```python
from build123d import *

# Parameters (mm, degrees)
SKETCH_1_W      = 20
SKETCH_1_H      = 52.5
SKETCH_1_R      = 3.1
EXTRUDE_1_DEPTH = 2
CHAMFER_1_SIZE  = 4
CHAMFER_2_SIZE  = 3


with BuildPart() as part:
    # 草图1 → 凸台-拉伸1 (new, symmetric)
    with BuildSketch(Plane.XY):
        Rectangle(SKETCH_1_W, SKETCH_1_H)
        with Locations((0, 16.25)):
            Circle(SKETCH_1_R, mode=Mode.SUBTRACT)
        with Locations((0, -3.75)):
            Circle(SKETCH_1_R, mode=Mode.SUBTRACT)
    extrude(amount=EXTRUDE_1_DEPTH, both=True)

    # 倒角1
    chamfer_1_edges = [part.edges().sort_by_distance(p)[0] for p in [
        (-10, 26.25, 0),
        (10, 26.25, 0),
        (10, -26.25, 0),
        (-10, -26.25, 0),
    ]]
    chamfer(chamfer_1_edges, length=CHAMFER_1_SIZE)

    # 倒角2
    chamfer_2_edges = [part.edges().sort_by_distance(p)[0] for p in [
        (-3.1, 16.25, 2),
        (-3.1, -3.75, 2),
    ]]
    chamfer(chamfer_2_edges, length=CHAMFER_2_SIZE)


solid = part.part
```
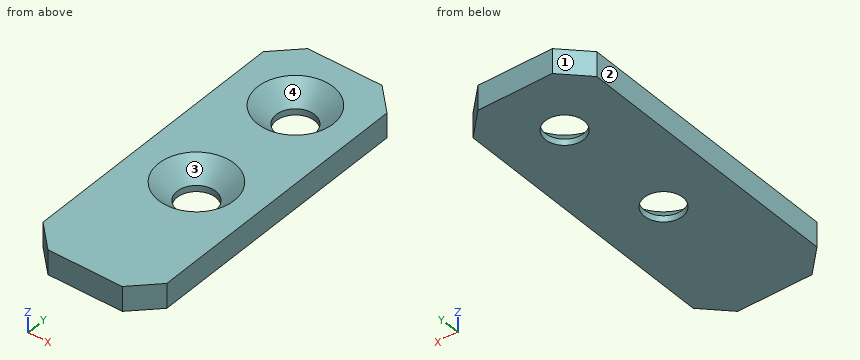
Build history of the part. All positions in model axes, mm. Face numbers are marked on the shaded views. Coordinates: 2 decimals unless noted, no trailing zeros. Order: outer loops, then holes, each group sorted by start corner. A loop starts at its lowest first (then second) coordinate and runs counter-clockwise, first axis right, second up. Notation, with made-up numbers: (57, -3.75) -> (101, -3.75) arc R5 ccw to (101, 4.25) -> close; hole circle Ø9 at (-17, -29). An arc over 180 degrees is marked (long way). Answer in a Markdown table with one row per item. Add a question column.
Q1. Band-saw the part on B-B, the plane x = 0. List the corners of the cut face in (y, z).
Q2. Wall check: line 1 along Y through (x, z) = (0, -1.8); line 2 along Y through (x, z) = (1.5, 0.85); line 3 along X through (y, z) = (17, -1.35). Give the ranges that are in metal, low to high. Write a range as [from, to].
Q3. Drop a flat-ended pin along its axis: pin 1 (2 mm diameter, centred on x = 7.5, z = 0, fed in from -Y). Give the stop position or say it passes through.
Q4. Band-saw the part on A-A, the plane y = 16.25. List the corners of the cut face in (x, z).
Q5. Band-saw the part on D-D, the plane x = -7.25. List the corners of the cut face in (y, z).
Q6. Band-saw the part on C-C, the plane z = 1. List the corners of the cut face in (x, y).
Q7. Mould opens along Y. For the marked faces 1, 2, 3 and 4 say: +Y half, -Y half, draft (parallel to the pull), parting line (faces both ways), or undercut.
Answers follow:
| question | item | result |
|---|---|---|
| 1 | outline | (-26.25, -2) -> (-6.85, -2) -> (-6.85, -1) -> (-9.85, 2) -> (-26.25, 2) -> close; (-0.65, -2) -> (13.15, -2) -> (13.15, -1) -> (10.15, 2) -> (2.35, 2) -> (-0.65, -1) -> close; (19.35, -2) -> (26.25, -2) -> (26.25, 2) -> (22.35, 2) -> (19.35, -1) -> close |
| 2 | line 1 | [-26.25, -6.85], [-0.65, 13.15], [19.35, 26.25] |
| 2 | line 2 | [-26.25, -8.47], [0.97, 11.53], [20.97, 26.25] |
| 2 | line 3 | [-10, -3.01], [3.01, 10] |
| 3 | pin 1 | y = -25.75 |
| 4 | outline | (-10, -2) -> (-3.1, -2) -> (-3.1, -1) -> (-6.1, 2) -> (-10, 2) -> close; (3.1, -2) -> (10, -2) -> (10, 2) -> (6.1, 2) -> (3.1, -1) -> close |
| 5 | outline | (-25, -2) -> (25, -2) -> (25, 2) -> (-25, 2) -> close |
| 6 | outline | (-10, -22.25) -> (-6, -26.25) -> (6, -26.25) -> (10, -22.25) -> (10, 22.25) -> (6, 26.25) -> (-6, 26.25) -> (-10, 22.25) -> close; hole circle Ø10.2 at (0, -3.75); hole circle Ø10.2 at (0, 16.25) |
| 7 | face 1 | +Y half |
| 7 | face 2 | draft |
| 7 | face 3 | undercut |
| 7 | face 4 | undercut |
